Here's the drawing with two shaded views (mm, measured from the low corner). I have some questions. Give positions to 0.01 mm unless a question says otherwise; leave off trailing zeros. Write each loop counter-clockwise with the first axis right and the second up, starting at its lowest first coordinate (ties: lowest second). Pieces come first, ordered by that corner, then holes. Notation, with made-up numbers: (-29, 31) -> (-4, 31) arc R33 ccw to (-4, 67) -> close; hole circle Ø8 at (-33.75, -13.5). An arc over 180 degrees is marked (long way). One line per item, written item: value.
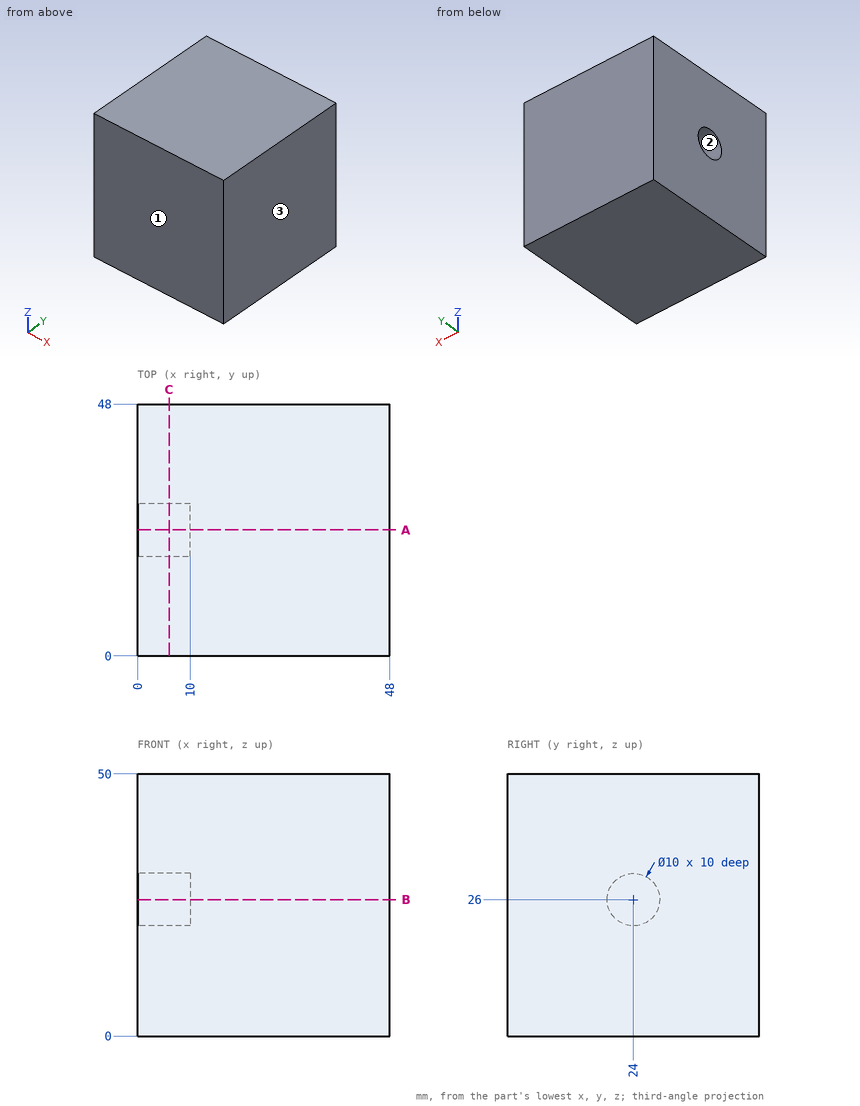
1) We'd pull the mould along Y, two halves only. Please class the marked faces 1, 2 and 3: released by +Y, released by -Y, zero draft, split by the parting line, or undercut.
Answer list:
face 1: released by -Y
face 2: undercut
face 3: zero draft
2) I need wall thicknesses on L1, parallel to Z at x = 5, y = 24. Which ranges of the line are inside material? Lowest first, please.
Answer list:
L1: z = 0 to 21, 31 to 50
3) If we section it at A-A (y = 24): Write out the boundary of the cut face in (x, z), and give its area (3 significant figures).
Answer list:
outline: (0, 0) -> (48, 0) -> (48, 50) -> (0, 50) -> (0, 31) -> (10, 31) -> (10, 21) -> (0, 21) -> close
area: 2,300 mm^2
4) Will this pin go through, and if not, where does the flat tip stop? pin 1 (3 mm diameter, centred on y = 25, z = 24, fed in from -X).
Answer list:
pin 1: stops at x = 10
5) If we section it at C-C (x = 6): Write out the boundary of the cut face in (y, z).
Answer list:
outline: (0, 0) -> (48, 0) -> (48, 50) -> (0, 50) -> close; hole circle Ø10 at (24, 26)
6) If we section it at B-B (z = 26): Write out the boundary of the cut face in (x, y).
Answer list:
outline: (0, 0) -> (48, 0) -> (48, 48) -> (0, 48) -> (0, 29) -> (10, 29) -> (10, 19) -> (0, 19) -> close
